```python
from build123d import *

# Parameters (mm, degrees)
SKETCH18_W              = 200.025
SKETCH18_H              = 139.7
BOSS_EXTRUDE6_DEPTH     = 25.4
SKETCH20_W              = 193.675
SKETCH20_H              = 139.7
CUT_EXTRUDE6_DEPTH      = 21.59
SKETCH22_W              = 200.025
SKETCH22_H              = 15.875
BOSS_EXTRUDE7_DEPTH     = 25.4
SKETCH23_W              = 200.025
SKETCH23_H              = 15.875
BOSS_EXTRUDE8_DEPTH     = 25.4
SKETCH24_W              = 168.275
SKETCH24_H              = 171.45
CUT_EXTRUDE7_DEPTH      = 3.175
SKETCH28_W              = 168.275
SKETCH28_H              = 12.7
CUT_EXTRUDE10_DEPTH     = 3.175
SKETCH31_R              = 1.65
SKETCH31_R_2            = 1.651
CUT_EXTRUDE15_DEPTH     = 1.825
CUT_EXTRUDE17_DEPTH     = 3.175
SKETCH39_R              = 2.2
CUT_EXTRUDE18_DEPTH     = 26.5
CUT_EXTRUDE20_DEPTH     = 5
SKETCH40_R              = 4.4
CUT_EXTRUDE19_DEPTH     = 17.225
SKETCH47_R              = 3.556
BOSS_EXTRUDE14_DEPTH    = 10.16
MIRROR6_COPY_1_SKETCH_R = 2.2
MIRROR6_COPY_1_DEPTH    = 26.5
MIRROR6_COPY_2_DEPTH    = 5
MIRROR6_COPY_3_SKETCH_R = 4.4
MIRROR6_COPY_3_DEPTH    = 17.225
CUT_EXTRUDE21_REACH     = 224.285
SKETCH48_R              = 6
SKETCH48_R_2            = 3.3
SKETCH48_R_3            = 2.75
SKETCH49_W              = 3.175
SKETCH49_H              = 93.98
BOSS_EXTRUDE15_DEPTH    = 6.35
SKETCH50_W              = 22.225
SKETCH50_H              = 3.175
BOSS_EXTRUDE16_DEPTH    = 19.05
FILLET1_R               = 6.35
FILLET2_R               = 3.175
FILLET3_R               = 12.7


with BuildPart() as part:
    # Sketch18 → Boss-Extrude6 (new body)
    with BuildSketch(Plane(origin=(0, 0, 0), x_dir=(1, 0, 0), z_dir=(0, 1, 0))):
        Rectangle(SKETCH18_W, SKETCH18_H)
    extrude(amount=BOSS_EXTRUDE6_DEPTH)

    # Sketch20 → Cut-Extrude6 (cut)
    with BuildSketch(Plane(origin=(0, 25.4, 0), x_dir=(1, 0, 0), z_dir=(0, 1, 0))):
        Rectangle(SKETCH20_W, SKETCH20_H)
    extrude(amount=-CUT_EXTRUDE6_DEPTH, mode=Mode.SUBTRACT)

    # Sketch22 → Boss-Extrude7 (add)
    with BuildSketch(Plane(origin=(0, 0, 0), x_dir=(1, 0, 0), z_dir=(0, 1, 0))):
        with Locations((0, -77.7875)):
            Rectangle(SKETCH22_W, SKETCH22_H)
    extrude(amount=BOSS_EXTRUDE7_DEPTH)

    # Sketch23 → Boss-Extrude8 (add)
    with BuildSketch(Plane(origin=(0, 0, 0), x_dir=(1, 0, 0), z_dir=(0, 1, 0))):
        with Locations((0, 77.7875)):
            Rectangle(SKETCH23_W, SKETCH23_H)
    extrude(amount=BOSS_EXTRUDE8_DEPTH)

    # Sketch24 → Cut-Extrude7 (cut)
    with BuildSketch(Plane(origin=(0, 25.4, 0), x_dir=(1, 0, 0), z_dir=(0, 1, 0))):
        Rectangle(SKETCH24_W, SKETCH24_H)
    extrude(amount=-CUT_EXTRUDE7_DEPTH, mode=Mode.SUBTRACT)

    # Sketch28 → Cut-Extrude10 (cut)
    with BuildSketch(Plane(origin=(0, 22.225, 0), x_dir=(1, 0, 0), z_dir=(0, 1, 0))):
        with Locations((0, 76.2)):
            Rectangle(SKETCH28_W, SKETCH28_H)
    cut_extrude10 = extrude(amount=-CUT_EXTRUDE10_DEPTH, mode=Mode.SUBTRACT)

    # Mirror5: Cut-Extrude10 across plane
    add(cut_extrude10.mirror(Plane.XY), mode=Mode.SUBTRACT)

    # Sketch31 → Cut-Extrude15 (cut)
    with BuildSketch(Plane(origin=(0, 3.81, 0), x_dir=(1, 0, 0), z_dir=(0, 1, 0))):
        with Locations(Location((-66.3575, 31.75, 0), (0, 0, 270))):
            Circle(SKETCH31_R)
        with Locations(Location((86.0425, 31.75, 0), (0, 0, 270))):
            Circle(SKETCH31_R_2)
        with Locations(Location((86.0425, -31.75, 0), (0, 0, 270))):
            Circle(SKETCH31_R_2)
        with Locations(Location((-66.3575, -31.75, 0), (0, 0, 270))):
            Circle(SKETCH31_R)
    extrude(amount=-CUT_EXTRUDE15_DEPTH, mode=Mode.SUBTRACT)

    # Sketch33 → Cut-Extrude17 (cut)
    with BuildSketch(Plane.XZ):
        Polygon((-63.5575, -33.366580754), (-63.5575, -30.133419246), (-66.3575, -28.516838493), (-69.1575, -30.133419246), (-69.1575, -33.366580754), (-66.3575, -34.983161507), align=None)
        Polygon((88.8425, -33.366580754), (88.8425, -30.133419246), (86.0425, -28.516838493), (83.2425, -30.133419246), (83.2425, -33.366580754), (86.0425, -34.983161507), align=None)
        Polygon((-63.5575, 33.366580754), (-66.3575, 34.983161507), (-69.1575, 33.366580754), (-69.1575, 30.133419246), (-66.3575, 28.516838493), (-63.5575, 30.133419246), align=None)
        Polygon((83.2425, 33.366580754), (83.2425, 30.133419246), (86.0425, 28.516838493), (88.8425, 30.133419246), (88.8425, 33.366580754), (86.0425, 34.983161507), align=None)
    extrude(amount=-CUT_EXTRUDE17_DEPTH, mode=Mode.SUBTRACT)

    # Sketch39 → Cut-Extrude18 (cut)
    with BuildSketch(Plane(origin=(0, 25.4, 0), x_dir=(1, 0, 0), z_dir=(0, 1, 0))):
        with Locations(Location((92.075, 77.7875, 0), (0, 0, 270))):
            Circle(SKETCH39_R)
    cut_extrude18 = extrude(amount=-CUT_EXTRUDE18_DEPTH, mode=Mode.SUBTRACT)

    # Sketch41 → Cut-Extrude20 (cut)
    with BuildSketch(Plane(origin=(0, 25.4, 0), x_dir=(1, 0, 0), z_dir=(0, 1, 0))):
        Polygon((89.996539031, 81.3875), (87.918078062, 77.7875), (89.996539031, 74.1875), (94.153460969, 74.1875), (96.231921938, 77.7875), (94.153460969, 81.3875), align=None)
    cut_extrude20 = extrude(amount=-CUT_EXTRUDE20_DEPTH, mode=Mode.SUBTRACT)

    # Sketch40 → Cut-Extrude19 (cut)
    with BuildSketch(Plane.XZ):
        with Locations(Location((92.075, -77.7875, 0), (0, 0, 270))):
            Circle(SKETCH40_R)
    cut_extrude19 = extrude(amount=-CUT_EXTRUDE19_DEPTH, mode=Mode.SUBTRACT)

    # Mirror3: Cut-Extrude18, Cut-Extrude20, Cut-Extrude19 across plane
    add(cut_extrude18.mirror(Plane.XY), mode=Mode.SUBTRACT)
    add(cut_extrude20.mirror(Plane.XY), mode=Mode.SUBTRACT)
    add(cut_extrude19.mirror(Plane.XY), mode=Mode.SUBTRACT)

    # Sketch47 → Boss-Extrude14 (add)
    # profile 1 of 2: a face of its own
    with BuildSketch(Plane.XZ):
        with BuildLine():
            Line((-44.45, -85.725), (-69.85, -85.725))
            ThreePointArc((-69.85, -85.725), (-65.589750808, -89.50934655), (-63.41304754, -94.775556275))
            ThreePointArc((-63.41304754, -94.775556275), (-61.253197141, -98.574568708), (-57.15, -100.078304866))
            ThreePointArc((-57.15, -100.078304866), (-53.046802859, -98.574568708), (-50.88695246, -94.775556275))
            ThreePointArc((-50.88695246, -94.775556275), (-48.710249192, -89.50934655), (-44.45, -85.725))
        make_face()
        with Locations(Location((-57.15, -93.728304866, 0), (0, 0, 270))):
            Circle(SKETCH47_R, mode=Mode.SUBTRACT)
    # profile 2 of 2: a face of its own
    with BuildSketch(Plane.XZ):
        with BuildLine():
            Line((69.85, -85.725), (44.45, -85.725))
            ThreePointArc((44.45, -85.725), (48.710249192, -89.50934655), (50.88695246, -94.775556275))
            ThreePointArc((50.88695246, -94.775556275), (53.046802859, -98.574568708), (57.15, -100.078304866))
            ThreePointArc((57.15, -100.078304866), (61.253197141, -98.574568708), (63.41304754, -94.775556275))
            ThreePointArc((63.41304754, -94.775556275), (65.589750808, -89.50934655), (69.85, -85.725))
        make_face()
        with Locations(Location((57.15, -93.728304866, 0), (0, 0, 270))):
            Circle(SKETCH47_R, mode=Mode.SUBTRACT)
    boss_extrude14 = extrude(amount=-BOSS_EXTRUDE14_DEPTH)

    # Mirror4: Boss-Extrude14 across plane
    add(boss_extrude14.mirror(Plane.XY))

    # Mirror6: Cut-Extrude18, Cut-Extrude20, Cut-Extrude19 across plane
    add(cut_extrude18.mirror(Plane(origin=(0, 0, 0), x_dir=(0, 0, 1), z_dir=(1, 0, 0))), mode=Mode.SUBTRACT)
    add(cut_extrude20.mirror(Plane(origin=(0, 0, 0), x_dir=(0, 0, 1), z_dir=(1, 0, 0))), mode=Mode.SUBTRACT)
    add(cut_extrude19.mirror(Plane(origin=(0, 0, 0), x_dir=(0, 0, 1), z_dir=(1, 0, 0))), mode=Mode.SUBTRACT)

    # Mirror6 copy 1 sketch → Mirror6 copy 1 (cut)
    with BuildSketch(Plane(origin=(0, 25.4, 0), x_dir=(-1, 0, 0), z_dir=(0, 1, 0))):
        with Locations(Location((92.075, 77.7875, 0), (0, 0, 270))):
            Circle(MIRROR6_COPY_1_SKETCH_R)
    extrude(amount=-MIRROR6_COPY_1_DEPTH, mode=Mode.SUBTRACT)

    # Mirror6 copy 2 sketch → Mirror6 copy 2 (cut)
    with BuildSketch(Plane(origin=(0, 25.4, 0), x_dir=(-1, 0, 0), z_dir=(0, 1, 0))):
        Polygon((89.996539031, 81.3875), (87.918078062, 77.7875), (89.996539031, 74.1875), (94.153460969, 74.1875), (96.231921938, 77.7875), (94.153460969, 81.3875), align=None)
    extrude(amount=-MIRROR6_COPY_2_DEPTH, mode=Mode.SUBTRACT)

    # Mirror6 copy 3 sketch → Mirror6 copy 3 (cut)
    with BuildSketch(Plane(origin=(0, 0, 0), x_dir=(-1, 0, 0), z_dir=(0, -1, 0))):
        with Locations(Location((92.075, -77.7875, 0), (0, 0, 270))):
            Circle(MIRROR6_COPY_3_SKETCH_R)
    extrude(amount=-MIRROR6_COPY_3_DEPTH, mode=Mode.SUBTRACT)

    # Sketch48 → Cut-Extrude21 (cut, up to next)
    with BuildSketch(Plane.ZY.offset(-96.8375), mode=Mode.PRIVATE) as cut_extrude21_sk1:
        with Locations((-60.325, 14.605)):
            Circle(SKETCH48_R)
    cut_extrude21_tool1 = extrude(cut_extrude21_sk1.sketch, amount=-CUT_EXTRUDE21_REACH, mode=Mode.PRIVATE) & part.part
    # Sketch48 → Cut-Extrude21 (cut, up to next)
    with BuildSketch(Plane.ZY.offset(-96.8375), mode=Mode.PRIVATE) as cut_extrude21_sk2:
        with Locations((60.325, 14.605)):
            Circle(SKETCH48_R_2)
    cut_extrude21_tool2 = extrude(cut_extrude21_sk2.sketch, amount=-CUT_EXTRUDE21_REACH, mode=Mode.PRIVATE) & part.part
    # Sketch48 → Cut-Extrude21 (cut, up to next)
    with BuildSketch(Plane.ZY.offset(-96.8375), mode=Mode.PRIVATE) as cut_extrude21_sk3:
        with Locations((-12.7, 17.78)):
            Circle(SKETCH48_R_3)
    cut_extrude21_tool3 = extrude(cut_extrude21_sk3.sketch, amount=-CUT_EXTRUDE21_REACH, mode=Mode.PRIVATE) & part.part
    # Sketch48 → Cut-Extrude21 (cut, up to next)
    with BuildSketch(Plane.ZY.offset(-96.8375), mode=Mode.PRIVATE) as cut_extrude21_sk4:
        with Locations((12.7, 17.78)):
            Circle(SKETCH48_R_3)
    cut_extrude21_tool4 = extrude(cut_extrude21_sk4.sketch, amount=-CUT_EXTRUDE21_REACH, mode=Mode.PRIVATE) & part.part
    add(cut_extrude21_tool1.solids().sort_by_distance((96.8375, 14.605, -60.325))[0], mode=Mode.SUBTRACT)
    add(cut_extrude21_tool2.solids().sort_by_distance((96.8375, 14.605, 60.325))[0], mode=Mode.SUBTRACT)
    add(cut_extrude21_tool3.solids().sort_by_distance((96.8375, 17.78, -12.7))[0], mode=Mode.SUBTRACT)
    add(cut_extrude21_tool4.solids().sort_by_distance((96.8375, 17.78, 12.7))[0], mode=Mode.SUBTRACT)

    # Sketch49 → Boss-Extrude15 (add)
    with BuildSketch(Plane(origin=(0, 3.81, 0), x_dir=(1, 0, 0), z_dir=(0, 1, 0))):
        with Locations((-76.2, 0)):
            Rectangle(SKETCH49_W, SKETCH49_H)
    extrude(amount=BOSS_EXTRUDE15_DEPTH)

    # Sketch50 → Boss-Extrude16 (add)
    with BuildSketch(Plane(origin=(0, 3.81, 0), x_dir=(1, 0, 0), z_dir=(0, 1, 0))):
        with Locations((-85.725, 48.5775)):
            Rectangle(SKETCH50_W, SKETCH50_H)
        with Locations((-85.725, -48.5775)):
            Rectangle(SKETCH50_W, SKETCH50_H)
    extrude(amount=BOSS_EXTRUDE16_DEPTH)

    # Fillet1
    fillet1_edges = [part.edges().sort_by_distance(p)[0] for p in [
        (100.0125, 12.7, 85.725),
        (-100.0125, 12.7, 85.725),
        (-100.0125, 12.7, -85.725),
        (100.0125, 12.7, -85.725),
    ]]
    fillet(fillet1_edges, radius=FILLET1_R)

    # Fillet2
    fillet2_edges = [part.edges().sort_by_distance(p)[0] for p in [
        (-96.8375, 3.81, -60.0075),
        (0, 3.81, -69.85),
        (0, 3.81, 69.85),
        (-74.6125, 3.81, 0),
        (-77.7875, 3.81, 0),
        (-96.8375, 3.81, 0),
        (-87.3125, 3.81, -46.99),
        (-85.725, 3.81, -50.165),
        (-96.8375, 3.81, 60.0075),
        (-87.3125, 3.81, 46.99),
        (-85.725, 3.81, 50.165),
    ]]
    fillet(fillet2_edges, radius=FILLET2_R)

    # Fillet3
    fillet3_edges = [part.edges().sort_by_distance(p)[0] for p in [
        (-76.2, 10.16, 46.99),
        (-76.2, 10.16, -46.99),
    ]]
    fillet(fillet3_edges, radius=FILLET3_R - 0.0001)  # a hair under: the kernel refuses the full size


solid = part.part
```
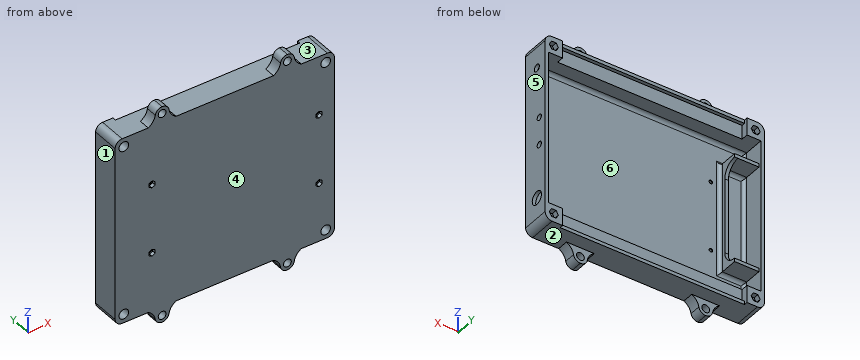
CAD build for the part. Positions are in the model's coordinates, mm. Face numbers are marked on the shaded views. A direction names the side the tool comes from. Give positions to 0.01 mm unless a question says otherwise; leave off trailing zeros. Loops run counter-clockwise (first coordinate to the right, second up) from the corner with the lowest first, then second, coordinate; pieces in that order, holes last. Notation, with made-up numbers: M 63.25,0.5 L 91.25,0.5 A25 ccw 91.25,17.5 Z; hole C -39.5,34.5 d3. An arc over 180 degrees is marked long. Use one line per item in the form item = value.
Item 1: Slice it at B-B (x = -5.5). List the corners of the cut face in (y, z) (3 decimals), plus the area to 3 significant figures.
Determined:
outline = M 0,-85.725 L 22.225,-85.725 L 22.225,-82.55 L 19.05,-82.55 L 19.05,-69.85 L 6.985,-69.85 A3.175 cw 3.81,-66.675 L 3.81,66.675 A3.175 cw 6.985,69.85 L 19.05,69.85 L 19.05,82.55 L 22.225,82.55 L 22.225,85.725 L 0,85.725 Z
area = 1,160 mm2
Item 2: Drill centre lines: probe 1 along X at (y, z) = (9, -1); probe 2 along X at (y, z) = (17, 74); probe 3 along Z at (x, y) = (-54, 19.5) (3 decimals). Where is each one in solid material? Low to high. Write a range as from..to.
Determined:
probe_1 = -100.01..-96.84, -77.79..-74.61, 96.84..100.01
probe_2 = -100.01..-94.31, -89.84..89.84, 94.31..100.01
probe_3 = -85.725..-82.55, 82.55..85.725
Item 3: Flat gauge pins, fed straight in: pin 1 (4 mm diameter, centred on x = 36, y = 2.5, fed in from -Z) (3 decimals); pin 2 (1.5 mm diameter, centred on x = -48.5, y = 7.5, fed in from +Z); pin 3 (2.5 mm diameter, centred on x = -76.5, z = -1.5, fed in from +Y). Where does each tip first touch, or does it go through?
Determined:
pin_1 = -85.725
pin_2 = 90.33
pin_3 = 10.16
Item 4: Which spindle directions (+Z, -Z, +X, -X, +Y, -Y) get a long thin tool onto all of the face, cutting with end or side? Do the marked faces 1, 2 and 3. Say none if no direction does.
Determined:
face_1 = +Z, -Z, -X, +Y, -Y
face_2 = -Z, +Y
face_3 = +Z, +Y
Item 5: Two-plate mould, pull along X, no slides. Class the marked faces 4, 5 and 6: pulls with the +X half, pulls with the -X half, needs draft (parallel to the pull), parting line crosses it, or undercut.
Determined:
face_4 = needs draft
face_5 = pulls with the +X half
face_6 = undercut
